Can you work these out from the model? Positions are in its coordinate system, mm. A direction names the side the tool comes from. Give positions to 0.01 mm unless a question says otherwise; leave off trailing zeros. Order: outer loops, then holes, each group sorted by start corner. A loop starts at its lowest first (then second) coordinate and runs counter-clockwise, first axis right, second up. Notation, with made-up numbers: (16, 86.25) -> (53, 86.25) arc R23 ccw to (53, 110.25) -> close; hole circle Ø5 at (81.5, 40.5). An arc over 180 degrees is marked (long way). Answer as a JSON object with one key per item and string values.
```python
from build123d import *


with BuildPart() as part:
    # Sketch1 → Base-Revolve (revolve)
    with BuildSketch(Plane.XY, mode=Mode.PRIVATE) as base_revolve_sk:
        with BuildLine():
            Line((0, 0), (5, 0))
            Line((5, 0), (5, 6.35))
            Line((5, 6.35), (7.5, 6.35))
            ThreePointArc((7.5, 6.35), (8.15921798, 9.167356917), (10, 11.399752469))
            Line((10, 11.399752469), (10, 21.35))
            ThreePointArc((10, 21.35), (4.672504387, 43.636025128), (8.888420475, 66.158795319))
            ThreePointArc((8.888420475, 66.158795319), (8.07243614, 75.409339174), (0, 80))
            Line((0, 80), (0, 0))
        make_face()
    revolve(base_revolve_sk.sketch.rotate(Axis((0, 0, 0), (0, -1, 0)), 90), axis=Axis((0, 0, 0), (0, -1, 0)))


solid = part.part
```
1. If we section it at B-B on y = 10: Please give me the cut outline in (x, z).
Worked answers:
{"outline": "circle Ø17.31 at (0, 0)"}
2. Please list where these lines run through material, in increasing order: L1, parallel to Z at x = 0.25, y = 15.5; L2, parallel to X at y = 17, z = 0.5; L3, parallel to X at y = 36, z = -2.75.
Worked answers:
{"L1": "-10 to 10", "L2": "-9.99 to 9.99", "L3": "-4.64 to 4.64"}
3. Will these pins go through, and if not, where does the flat tip stop? pin 1 Ø8 at (y, z) = (52, -1.5) entering from -X; pin 2 Ø1 at (x, y) = (-5.5, 40) entering from -Z (3 decimals); pin 3 Ø5 at (x, y) = (-5, 9.5) entering from +Z; pin 4 Ø4 at (x, z) = (2.5, 7) entering from +Y.
Worked answers:
{"pin 1": "x = -5.72", "pin 2": "through", "pin 3": "z = 9.41", "pin 4": "y = 78.17"}
4. If we section it at A-A on y = 41: Please give me the cut outline in (x, z).
Worked answers:
{"outline": "circle Ø9.6 at (0, 0)"}
5. For faces 1 (the face through (0, 0, 0)), 2 (the face through (0, 3, -5)), which set-ups out of +Z, -Z, +X, -X, +Y, -Y let a thin tool reach every point of the face, with its end or its side?
Worked answers:
{"face 1": "+Z, -Z, +X, -X, -Y", "face 2": "-Y"}
